from build123d import *

# Parameters (mm, degrees)
F1_DEPTH = 25.4
F2_R     = 23.0115173136
F3_DEPTH = 20.066
F5_DEPTH = 65.533


with BuildPart() as f1:
    # F0 (on Front) → F1 (new body)
    with BuildSketch(Plane.XZ):
        with BuildLine():
            Line((23.2431292534, -60.0447505713), (23.2431292534, 60.0447505713))
            ThreePointArc((23.2431292534, 60.0447505713), (0, 36.8016213179), (-23.2431292534, 60.0447505713))
            Line((-23.2431292534, 60.0447505713), (-23.2431292534, -60.0447505713))
            Line((-23.2431292534, -60.0447505713), (-22.8073433001, -60.0447505713))
            ThreePointArc((-22.8073433001, -60.0447505713), (0, -37.2374072712), (22.8073433001, -60.0447505713))
            Line((22.8073433001, -60.0447505713), (23.2431292534, -60.0447505713))
        make_face()
        with BuildLine():
            Line((23.2431292534, 60.0447505713), (13.2014414659, 60.0447505713))
            ThreePointArc((13.2014414659, 60.0447505713), (0, 46.8433091053), (-13.2014414659, 60.0447505713))
            Line((-13.2014414659, 60.0447505713), (-23.2431292534, 60.0447505713))
            ThreePointArc((-23.2431292534, 60.0447505713), (0, 36.8016213179), (23.2431292534, 60.0447505713))
        make_face()
        with BuildLine():
            Line((12.0115778455, -60.0447505713), (22.8073433001, -60.0447505713))
            ThreePointArc((22.8073433001, -60.0447505713), (0, -37.2374072712), (-22.8073433001, -60.0447505713))
            Line((-22.8073433001, -60.0447505713), (-12.0115778455, -60.0447505713))
            ThreePointArc((-12.0115778455, -60.0447505713), (0, -48.0331727257), (12.0115778455, -60.0447505713))
        make_face()
        with BuildLine():
            ThreePointArc((-22.8073433001, -60.0447505713), (0, -82.8520938713), (22.8073433001, -60.0447505713))
            Line((22.8073433001, -60.0447505713), (12.0115778455, -60.0447505713))
            ThreePointArc((12.0115778455, -60.0447505713), (0, -72.0563284168), (-12.0115778455, -60.0447505713))
            Line((-12.0115778455, -60.0447505713), (-22.8073433001, -60.0447505713))
        make_face()
        with BuildLine():
            ThreePointArc((-13.2014414659, 60.0447505713), (0, 73.2461920372), (13.2014414659, 60.0447505713))
            Line((13.2014414659, 60.0447505713), (23.2431292534, 60.0447505713))
            ThreePointArc((23.2431292534, 60.0447505713), (0, 83.2878798246), (-23.2431292534, 60.0447505713))
            Line((-23.2431292534, 60.0447505713), (-13.2014414659, 60.0447505713))
        make_face()
    extrude(amount=F1_DEPTH)

    # F2 (on face) → F3 (join)
    with BuildSketch(Plane(origin=(0, 0, 0), x_dir=(-1, 0, 0), z_dir=(0, 1, 0))):
        with Locations((0, -60.0447505713)):
            Circle(F2_R)
    extrude(amount=F3_DEPTH)

    # F4: F1 across face


with BuildPart() as f1_1:
    add(f1.part)
    add(f1.part.mirror(Plane(origin=(0, 20.066, -60.0447505713), x_dir=(-1, 0, 0), z_dir=(0, 1, 0))))

    # F5 (cut, through all): a face of the model
    f5_faces = [f1_1.faces().sort_by_distance(p)[0] for p in [
        (0, 0, -60.0447505713),
    ]]
    extrude(f5_faces, amount=-F5_DEPTH, mode=Mode.SUBTRACT)


solid = f1_1.part
For this review, take the finished solid that the model builds, in its own axes (mm). A direction names the side the tool comes from. Give positions to 0.01 mm unless a question says otherwise; leave off trailing zeros. Loops run counter-clockwise (first coordinate to the right, second up) from the corner with the lowest first, then second, coordinate; pieces in that order, holes last.
Item 1: Take a section at C-C, the plane y = -16. State the section outline as (x, z) points.
Item 2: Take a section at B-B, the plane x = 0. State the section outline as (y, z) points, and give its area (3 significant figures).
Item 3: Tool access review of faces 5 (the cylindrical face through (-0.502, 52.654, -82.847)), 6 (the cylindrical face through (0.511, -12.522, 83.282)), 7 (the cylindrical face through (-0.502, -12.522, -82.847)): name each direction out of +Z, -Z, +X, -X, +Y, -Y from which nothing blocks a thin tool from reaching the whole face with its end or side.
Item 4: Take a section at A-A, the plane z = -32. State the section outline as (x, y) points.
Item 5: Insertion check: pin 1 (1.5 mm diameter, centred on y = 2, z = -56.5, fed in from +X); pin 2 (5 mm diameter, centred on x = 2, y = 7.5, fed in from +Z); pin 3 (1 mm diameter, centred on x = 4.5, y = 52.5, fed in from +Z). Each pin has a flat end and moves straight along its axis. Give the tip position at first contact, or say it passes through.
Item 6: For line 1 along Z through (x, y) = (0, -6.5); line 2 along Y through (x, z) = (15.5, 60); line 3 along Z through (x, y) = (8.5, 46.5), list the stretches that pass through material, from the lowest coordinate up.
Item 7: Draft analysis for pull direction Y (two halves, no side actions). For faces 1 (the flat face through (23.243, 53, -1)), 2 (the flat face through (0, 40.132, 13)), 3 (the cylindrical face through (4.99, 20.35, -82.51)), 4 (the flat face through (0, -25.4, 1)), state which applies: +Y half, -Y half, draft (parallel to the pull), parting line (faces both ways), or undercut.
Item 8: Take a section at D-D, the plane x = -20. State the section outline as (y, z) points, and give its area (3 significant figures).
Calculated:
1. outline: (-23.24, -60.04) - (-22.81, -60.04) arc R22.81 ccw to (22.81, -60.04) - (23.24, -60.04) - (23.24, 60.04) arc R23.24 ccw to (-23.24, 60.04) - close; hole circle Ø26.4 at (0, 60.04); hole circle Ø24.02 at (0, -60.04)
2. outline: (-25.4, -82.85) - (0, -82.85) - (0, -83.06) - (40.13, -83.06) - (40.13, -82.85) - (65.53, -82.85) - (65.53, -72.06) - (-25.4, -72.06) - close; (-25.4, -48.03) - (65.53, -48.03) - (65.53, 46.84) - (40.13, 46.84) - (40.13, -37.03) - (0, -37.03) - (0, 46.84) - (-25.4, 46.84) - close; (-25.4, 73.25) - (0, 73.25) - (0, 83.29) - (-25.4, 83.29) - close; (40.13, 73.25) - (65.53, 73.25) - (65.53, 83.29) - (40.13, 83.29) - close
2. area: 6,760 mm2
3. face 5: -Z, +Y
3. face 6: +Z, +Y, -Y
3. face 7: -Z, -Y
4. outline: (-23.24, -25.4) - (23.24, -25.4) - (23.24, 0) - (-23.24, 0) - close; (-23.24, 40.13) - (23.24, 40.13) - (23.24, 65.53) - (-23.24, 65.53) - close
5. pin 1: stops at x = 22.84
5. pin 2: stops at z = -37.03
5. pin 3: stops at z = 82.94
6. line 1: z = -82.85 to -72.06, -48.03 to 46.84, 73.25 to 83.29
6. line 2: y = -25.4 to 0, 40.13 to 65.53
6. line 3: z = -81.21 to -68.53, -51.56 to 49.94, 70.15 to 81.68
7. face 1: draft
7. face 2: undercut
7. face 3: undercut
7. face 4: -Y half
8. outline: (-25.4, -71.01) - (0, -71.01) - (0, -71.43) - (40.13, -71.43) - (40.13, -71.01) - (65.53, -71.01) - (65.53, 71.89) - (40.13, 71.89) - (40.13, -48.66) - (0, -48.66) - (0, 71.89) - (-25.4, 71.89) - close
8. area: 8,170 mm2
